Model file for the job. Use its own axes, mm. Face numbers are marked on the shaded views. A direction names the side the tool comes from. Round coordinates to 2 decimals unless told otherwise and drop trailing zeros. Loops run counter-clockwise (first coordinate to the right, second up) from the corner with the lowest first, then second, coordinate; pieces in that order, holes last. Notation, with made-up numbers: M 36,25 L 44,25 A27 ccw 44,43 Z; hole C 58.25,53 d3. An arc over 180 degrees is marked long. Use a Markdown table: item, result. Add a question column.
Item 1: Saw through at C-C on z = 1.45. Write the cut outline in (x, y), then the cut area to 3 significant figures.
Item 2: Two-plate mould, pull along Y, no slides. Class the marked faces 1, 2, 3 and 4: +Y half, -Y half, draft (parallel to the pull), parting line (faces both ways), or undercut.
Item 3: Pin check, flat tips, straight feed: P1, Ø7.5, axis at x = 2.5, y = 6.5, coming from the +Z side; P2, Ø0.9, axis at x = 6.5, z = 3.5, coming from the -Y side. Stop position of each tip, or through.
Item 4: Tool access for the marked faces 5, 6, 7, 8 and 9: list every direction of +Z, -Z, +X, -X, +Y, -Y with a clear straight run to the whole face (end or side of a thin tool).
Item 5: Saw through at A-A on x = 0. Write the cut outline in (y, z).
Item 6: Saw through at B-B on y = 7.25. Write the cut outline in (x, z), then the cut area to 3 significant figures.
Item 7: Wall check: L1, parallel to X at y = 8, z = 3.75; L2, parallel to Z at x = 5, y = 12; L3, parallel to X at y = 9.25, z = 2.35. Give the ranges that are in metal, low to high. Write a range as from..to.
Item 8: Saw through at D-D on y = 12.5. Write the cut outline in (x, z).
```python
from build123d import *

# Parameters (mm, degrees)
EXTRUDE_1_DEPTH = 3
SKETCH_2_W      = 1.8
SKETCH_2_H      = 6
EXTRUDE_2_DEPTH = 2.1


with BuildPart() as part:
    # Эскиз1 → Бобышка-Вытянуть1 (new body)
    with BuildSketch(Plane.XY):
        with BuildLine():
            Line((-7.7, 13.737499607), (7.7, 13.737499607))
            Line((7.7, 13.737499607), (7.7, -0.039604792))
            Line((7.7, -0.039604792), (7.7, -2.309398114))
            Line((7.7, -2.309398114), (2.10443313, -2.309398114))
            ThreePointArc((2.10443313, -2.309398114), (0, -1.158976271), (-2.10443313, -2.309398114))
            Line((-2.10443313, -2.309398114), (-7.7, -2.309398114))
            Line((-7.7, -2.309398114), (-7.7, -0.039604792))
            Line((-7.7, -0.039604792), (-7.7, 13.737499607))
        make_face()
        with BuildLine():
            Line((4, 7.737499607), (4, 5.041023729))
            ThreePointArc((4, 5.041023729), (0, 1.041023729), (-4, 5.041023729))
            Line((-4, 5.041023729), (-4, 7.737499607))
            ThreePointArc((-4, 7.737499607), (0, 11.737499607), (4, 7.737499607))
        make_face(mode=Mode.SUBTRACT)
    extrude(amount=EXTRUDE_1_DEPTH)

    # Эскиз2 → Бобышка-Вытянуть2 (add)
    with BuildSketch(Plane.XY.offset(3)):
        with Locations((-6.8, 10.737499607)):
            Rectangle(SKETCH_2_W, SKETCH_2_H)
        with Locations((6.8, 10.737499607)):
            Rectangle(SKETCH_2_W, SKETCH_2_H)
    extrude(amount=EXTRUDE_2_DEPTH)


solid = part.part
```
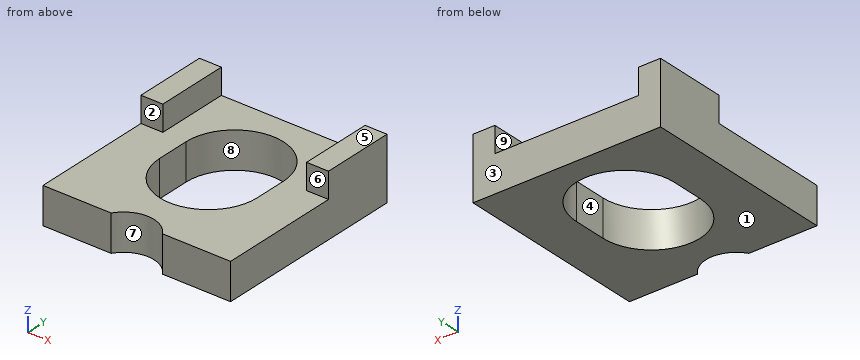
Entries:
| question | item | result |
|---|---|---|
| 1 | outline | M -7.7,-2.31 L -2.1,-2.31 A2.5 cw 2.1,-2.31 L 7.7,-2.31 L 7.7,13.74 L -7.7,13.74 Z; hole M -4,5.04 A4 ccw 4,5.04 L 4,7.74 A4 ccw -4,7.74 Z |
| 1 | area | 172 mm2 |
| 2 | face 1 | draft |
| 2 | face 2 | -Y half |
| 2 | face 3 | +Y half |
| 2 | face 4 | undercut |
| 3 | P1 | z = 5.1 |
| 3 | P2 | y = 7.74 |
| 4 | face 5 | +Z, +X, -X, +Y, -Y |
| 4 | face 6 | +Z, +X, -X, -Y |
| 4 | face 7 | +Z, -Z, -Y |
| 4 | face 8 | +Z, -Z |
| 4 | face 9 | +Z, +Y, -Y |
| 5 | outline | M -1.16,0 L 1.04,0 L 1.04,3 L -1.16,3 Z; M 11.74,0 L 13.74,0 L 13.74,3 L 11.74,3 Z |
| 6 | outline | M -7.7,0 L -4,0 L -4,3 L -7.7,3 Z; M 4,0 L 7.7,0 L 7.7,3 L 4,3 Z |
| 6 | area | 22.2 mm2 |
| 7 | L1 | -7.7..-5.9, 5.9..7.7 |
| 7 | L2 | 0..3 |
| 7 | L3 | -7.7..-3.7, 3.7..7.7 |
| 8 | outline | M -7.7,0 L 7.7,0 L 7.7,5.1 L 5.9,5.1 L 5.9,3 L -5.9,3 L -5.9,5.1 L -7.7,5.1 Z |
